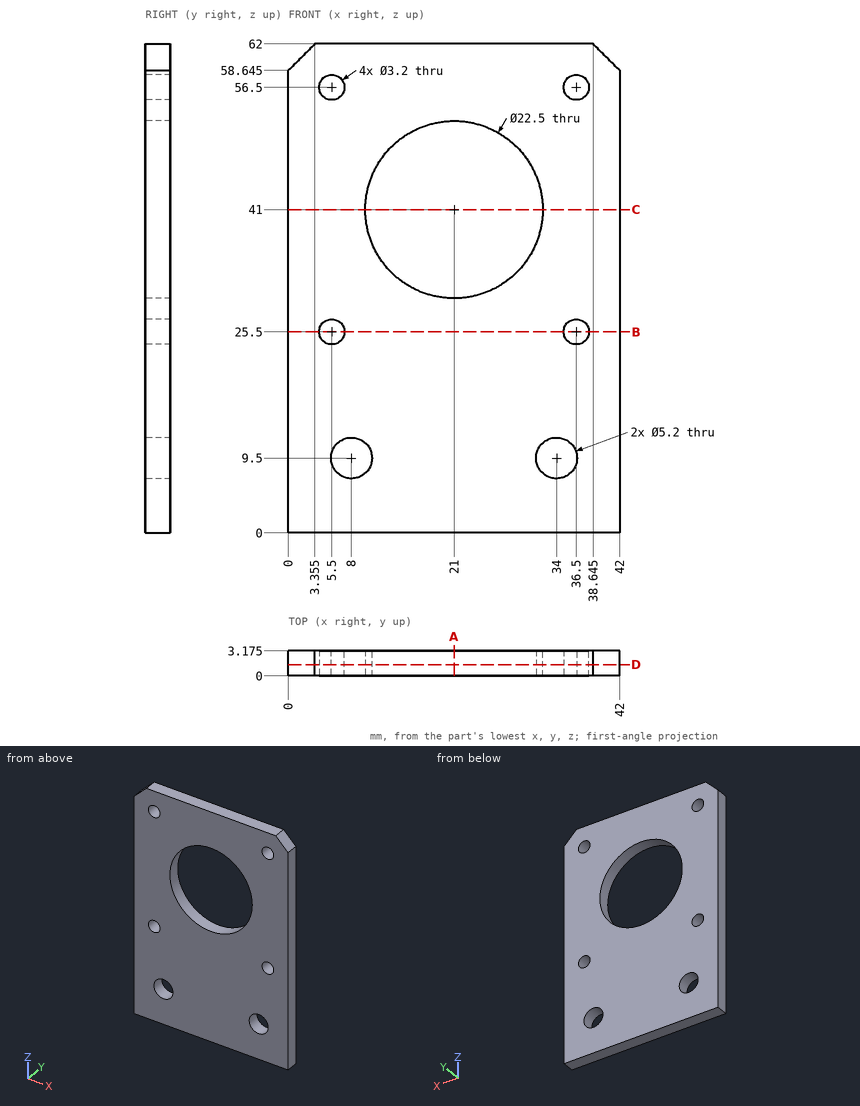
Drawing for the job (mm, zero at the part's lowest x, y, z). Round coordinates to 2 decimals unless told otherwise and drop trailing zeros. Write each loop counter-clockwise with the first axis right and the second up, starting at its lowest first coordinate (ties: lowest second). Pieces come first, ordered by that corner, then holes. Notation, with made-up numbers: (28.5, 13) - (79.5, 13) arc R25 ccw to (79.5, 29) - close; hole circle Ø6 at (58.25, 21). An arc over 180 degrees is marked (long way). Write item = value, one per line. Start each with the question number.
Q1. Band-saw the part on B-B (z = 25.5). Give the cut face in (x, y) (3 decimals), then the cut area to 3 significant figures.
Q2. Band-saw the part on A-A (x = 21). Give the cut face in (y, z) (3 decimals), then the cut area to 3 significant figures.
Q3. Drop a flat-ended pin along its axis: pin 1 (3 mm diameter, centred on x = 5.5, z = 25.5, fed in from +Y). Give the stop position or say it passes through.
Q4. Probe L1, parallel to X at y = 1, z = 25.5; L2, parallel to Z at x = 37, y = 0.7; L3, parallel to Z at x = 34, y = 2.1. List the from-to ranges inside material, lowest first. Write a range as from..to.
Q5. Band-saw the part on D-D (y = 1.45). Give the cut face in (x, z) (3 decimals).
Q6. Band-saw the part on C-C (z = 41). Give the cut face in (x, y) (3 decimals), then the cut area to 3 significant figures.
Answers below:
q1.outline = (0, 0) - (3.9, 0) - (3.9, 3.175) - (0, 3.175) - close; (7.1, 0) - (34.9, 0) - (34.9, 3.175) - (7.1, 3.175) - close; (38.1, 0) - (42, 0) - (42, 3.175) - (38.1, 3.175) - close
q1.area = 113 mm2
q2.outline = (0, 0) - (3.175, 0) - (3.175, 29.75) - (0, 29.75) - close; (0, 52.25) - (3.175, 52.25) - (3.175, 62) - (0, 62) - close
q2.area = 125 mm2
q3.pin_1 = through
q4.L1 = 0..3.9, 7.1..34.9, 38.1..42
q4.L2 = 0..23.98, 27.02..54.98, 58.02..62
q4.L3 = 0..6.9, 12.1..62
q5.outline = (0, 0) - (42, 0) - (42, 58.645) - (38.645, 62) - (3.355, 62) - (0, 58.645) - close; hole circle Ø3.2 at (5.5, 25.5); hole circle Ø3.2 at (5.5, 56.5); hole circle Ø5.2 at (8, 9.5); hole circle Ø22.5 at (21, 41); hole circle Ø5.2 at (34, 9.5); hole circle Ø3.2 at (36.5, 25.5); hole circle Ø3.2 at (36.5, 56.5)
q6.outline = (0, 0) - (9.75, 0) - (9.75, 3.175) - (0, 3.175) - close; (32.25, 0) - (42, 0) - (42, 3.175) - (32.25, 3.175) - close
q6.area = 61.9 mm2
